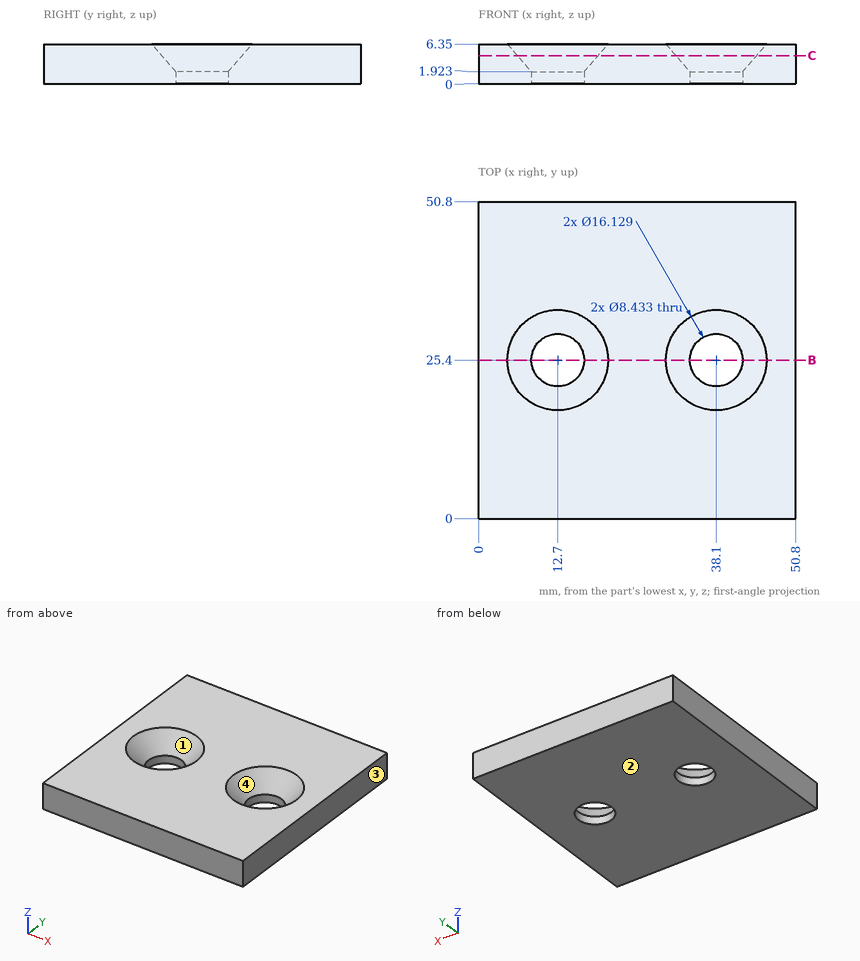
Geometry check sheet. Reference: drawing and pictorial views, mm from the part's lowest x, y, z. Give positions to 0.01 mm unless a question says otherwise; leave off trailing zeros. Loops run counter-clockwise (first coordinate to the right, second up) from the corner with the lowest first, then second, coordinate; pieces in that order, holes last. Notation, with made-up numbers: (27.5, 85.5) -> (64.5, 85.5) arc R25 cw to (64.5, 119.5) -> close; hole circle Ø9 at (-28, -13.5). An arc over 180 degrees is marked (long way). Answer in a Markdown table with one row per item. Add a question column.
1) Cross-section at B-B on y = 25.4. State how many separate pieces and enclosed holes the cut face has, and give its area (3 significant figures).
2) Material ranges on probe 1 along X at (y, z) = (25.4, 1.2); probe 2 along X at (y, z) = (22.5, 2.75); probe 3 along Y at (x, z) = (38.1, 1.35), recorded low to high. Write a range as from..to.
3) Gauge pin test, flat end, axial feed: P1, Ø2, axis at x = 44.5, y = 18, coming from the -Z side. Record the tip position at first contact, or that the pin passes through.
4) Draft check along X on the marked faces 1, 2, 3 and 4. Enter one of: pulls with the +X half, pulls with the -X half, needs draft (parallel to the pull), parting line crosses it, or undercut.
5) Cross-section at C-C on z = 4.5. Record the boundary of the cut face in (x, y), and give its area (3 significant figures).
Outcome:
| question | item | result |
|---|---|---|
| 1 | separate pieces | 3 |
| 1 | enclosed holes | 0 |
| 1 | area | 181 mm^2 |
| 2 | probe 1 | x = 0..8.48, 16.92..33.88, 42.32..50.8 |
| 2 | probe 2 | x = 0..8.71, 16.69..34.11, 42.09..50.8 |
| 2 | probe 3 | y = 0..21.18, 29.62..50.8 |
| 3 | P1 | stops at z = 0 |
| 4 | face 1 | undercut |
| 4 | face 2 | needs draft |
| 4 | face 3 | pulls with the +X half |
| 4 | face 4 | undercut |
| 5 | outline | (0, 0) -> (50.8, 0) -> (50.8, 50.8) -> (0, 50.8) -> close; hole circle Ø12.91 at (12.7, 25.4); hole circle Ø12.91 at (38.1, 25.4) |
| 5 | area | 2,320 mm^2 |
